```python
from build123d import *

# Parameters (mm, degrees)
BOSS_EXTRUDE1_DEPTH = 6.35
SKETCH2_R           = 1.1303
CUT_EXTRUDE1_DEPTH  = 7.9375
FILLET1_R           = 0.762


with BuildPart() as part:
    # Sketch1 → Boss-Extrude1 (new body)
    with BuildSketch(Plane(origin=(0, 0, 0), x_dir=(1, 0, 0), z_dir=(0, 1, 0))):
        Polygon((0, 7.9375), (4.953, 7.9375), (4.953, 3.175), (9.017, 3.175), (9.017, 7.9375), (13.97, 7.9375), (13.97, 0), (0, 0), align=None)
    extrude(amount=BOSS_EXTRUDE1_DEPTH)

    # Sketch2 → Cut-Extrude1 (cut)
    with BuildSketch(Plane.XY):
        with Locations((2.413, 3.175)):
            Circle(SKETCH2_R)
        with Locations((11.557, 3.175)):
            Circle(SKETCH2_R)
    extrude(amount=-CUT_EXTRUDE1_DEPTH, mode=Mode.SUBTRACT)

    # Fillet1
    fillet1_edges = [part.edges().sort_by_distance(p)[0] for p in [
        (13.97, 6.35, -3.96875),
        (6.985, 0, 0),
        (0, 0, -3.96875),
        (11.4935, 6.35, -7.9375),
        (0, 3.175, -7.9375),
        (4.953, 3.175, -7.9375),
        (9.017, 3.175, -7.9375),
        (13.97, 3.175, -7.9375),
        (13.97, 3.175, 0),
        (0, 3.175, 0),
        (9.017, 6.35, -5.55625),
        (6.985, 6.35, -3.175),
        (4.953, 6.35, -5.55625),
        (2.4765, 6.35, -7.9375),
        (0, 6.35, -3.96875),
        (6.985, 6.35, 0),
        (2.4765, 0, -7.9375),
        (4.953, 0, -5.55625),
        (6.985, 0, -3.175),
        (9.017, 0, -5.55625),
        (11.4935, 0, -7.9375),
        (13.97, 0, -3.96875),
    ]]
    fillet(fillet1_edges, radius=FILLET1_R)


solid = part.part
```
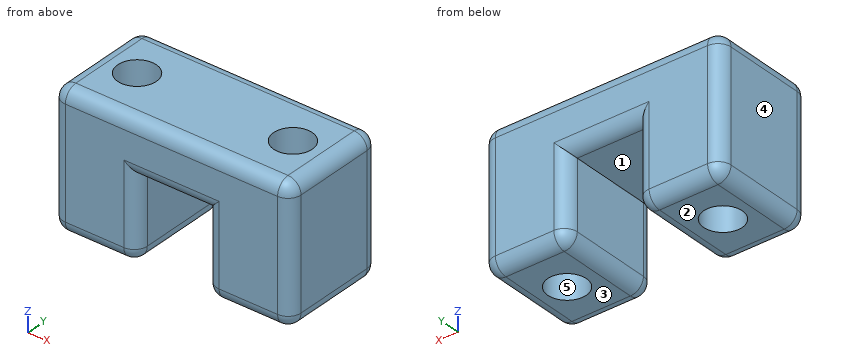
Model file for the job. Use its own axes, mm. Face numbers are marked on the shaded views. A direction names the side the tool comes from. Give positions to 0.01 mm unless a question says otherwise; leave off trailing zeros. Order: outer loops, then holes, each group sorted by start corner. A loop starts at its lowest first (then second) coordinate and runs counter-clockwise, first axis right, second up.
1) Saw through at B-B, the plane x = 3.25. Write the cut outline in (y, z).
2) Pin check, flat tips, straight feed: pin 1 (1 mm diameter, centred on x = 6.5, y = 1.5, fed in from -Z) (3 decimals); pin 2 (1.4 mm diameter, centred on x = 11.557, y = 3.175, fed in from -Z). Stop position of each tip, or through.
3) Saw through at A-A, the plane z = -6.25. Write the cut outline in (x, y) (3 decimals).
4) Saw through at D-D, the plane z = -1.75. Write the cut outline in (x, y) (3 decimals), then the cut area to 3 significant figures.
5) Mould opens along X. For the marked faces 3, 4 and 5 say: +X half, -X half, draft (parallel to the pull), parting line (faces both ways), or undercut.
6) Saw through at C-C, the plane y = 4. Write the cut outline in (x, z) (1 decimal).
7) Wall check: probe 1 along X at (y, z) = (1.25, -5.5); probe 2 along X at (y, z) = (3.25, -7.25); probe 3 along X at (y, z) = (4, -7.5). Give the ranges that are in metal, low to high.
8) 3-axis set-ups, long thin cutter, end or side, ignore diameter. For the marked faces 1 and 2: which of +Z, -Z, +X, -X, +Y, -Y reach the whole face in a straight line?
Computed:
1. outline: (0, -7.18) arc R0.76 ccw to (0.76, -7.94) - (2.42, -7.94) - (2.42, 0) - (0.76, 0) arc R0.76 ccw to (0, -0.76) - close; (3.93, -7.94) - (5.59, -7.94) arc R0.76 ccw to (6.35, -7.18) - (6.35, -0.76) arc R0.76 ccw to (5.59, 0) - (3.93, 0) - close
2. pin 1: stops at z = -3.175
2. pin 2: passes through
3. outline: (0, 0.762) arc R0.762 ccw to (0.762, 0) - (4.191, 0) arc R0.762 ccw to (4.953, 0.762) - (4.953, 5.588) arc R0.762 ccw to (4.191, 6.35) - (0.762, 6.35) arc R0.762 ccw to (0, 5.588) - close; (9.017, 0.762) arc R0.762 ccw to (9.779, 0) - (13.208, 0) arc R0.762 ccw to (13.97, 0.762) - (13.97, 5.588) arc R0.762 ccw to (13.208, 6.35) - (9.779, 6.35) arc R0.762 ccw to (9.017, 5.588) - close; hole circle Ø2.261 at (2.413, 3.175); hole circle Ø2.261 at (11.557, 3.175)
4. outline: (0, 0.762) arc R0.762 ccw to (0.762, 0) - (13.208, 0) arc R0.762 ccw to (13.97, 0.762) - (13.97, 5.588) arc R0.762 ccw to (13.208, 6.35) - (0.762, 6.35) arc R0.762 ccw to (0, 5.588) - close; hole circle Ø2.261 at (2.413, 3.175); hole circle Ø2.261 at (11.557, 3.175)
4. area: 80.2 mm2
5. face 3: draft
5. face 4: -X half
5. face 5: undercut
6. outline: (0, -7.2) arc R0.8 ccw to (0.8, -7.9) - (1.6, -7.9) - (1.6, 0) - (0.8, 0) arc R0.8 ccw to (0, -0.8) - close; (3.2, -7.9) - (4.2, -7.9) arc R0.8 ccw to (5, -7.2) - (5, -3.2) - (9, -3.2) - (9, -7.2) arc R0.8 ccw to (9.8, -7.9) - (10.8, -7.9) - (10.8, 0) - (3.2, 0) - close; (12.3, -7.9) - (13.2, -7.9) arc R0.8 ccw to (14, -7.2) - (14, -0.8) arc R0.8 ccw to (13.2, 0) - (12.3, 0) - close
7. probe 1: x = 0 to 4.95, 9.02 to 13.97
7. probe 2: x = 0 to 1.29, 3.54 to 4.95, 9.02 to 10.43, 12.68 to 13.97
7. probe 3: x = 0.07 to 1.64, 3.19 to 4.88, 9.09 to 10.78, 12.33 to 13.9
8. face 1: -Z, +Y, -Y
8. face 2: -Z, +X, -X, +Y, -Y
